```python
from build123d import *

# Parameters (mm, degrees)
SKETCH1_W                      = 57.404
SKETCH1_H                      = 61.214
BOSS_EXTRUDE1_DEPTH            = 1.5875
BOSS_EXTRUDE2_DEPTH            = 1.5875
BOSS_EXTRUDE3_DEPTH            = 54.229
BOSS_EXTRUDE4_DEPTH            = 1.5875
SKETCH6_W                      = 1.63195
SKETCH6_H                      = 1.5875
F_4_CLEARANCE_HOLE1_AT_2_COUNT = 2
F_4_CLEARANCE_HOLE1_AT_2_PITCH = 54.864


with BuildPart() as part:
    # Sketch1 → Boss-Extrude1 (new body)
    with BuildSketch(Plane(origin=(0, 0, 0), x_dir=(1, 0, 0), z_dir=(0, 1, 0))):
        with Locations((28.702, -30.607)):
            Rectangle(SKETCH1_W, SKETCH1_H)
    extrude(amount=BOSS_EXTRUDE1_DEPTH)

    # Sketch2 → Boss-Extrude2 (add)
    with BuildSketch(Plane(origin=(57.404, 0, 0), x_dir=(0, 0, -1), z_dir=(1, 0, 0))):
        with BuildLine():
            Line((-61.214, 1.5875), (0, 1.5875))
            Line((0, 1.5875), (0, 9.144))
            ThreePointArc((0, 9.144), (-1.859871939, 13.634128061), (-6.35, 15.494))
            Line((-6.35, 15.494), (-54.864, 15.494))
            ThreePointArc((-54.864, 15.494), (-59.354128061, 13.634128061), (-61.214, 9.144))
            Line((-61.214, 9.144), (-61.214, 1.5875))
        make_face()
    extrude(amount=-BOSS_EXTRUDE2_DEPTH)

    # Sketch3 → Boss-Extrude3 (add)
    with BuildSketch(Plane.ZY.offset(-55.8165)):
        with BuildLine():
            Line((1.5875, 1.5875), (1.5875, 3.175))
            Line((1.5875, 3.175), (1.5875, 9.144))
            ThreePointArc((1.5875, 9.144), (2.982403955, 12.511596045), (6.35, 13.9065))
            Line((6.35, 13.9065), (6.35, 15.494))
            ThreePointArc((6.35, 15.494), (1.859871939, 13.634128061), (0, 9.144))
            Line((0, 9.144), (0, 1.5875))
            Line((0, 1.5875), (1.5875, 1.5875))
        make_face()
        with BuildLine():
            Line((59.6265, 9.144), (59.6265, 3.175))
            Line((59.6265, 3.175), (59.6265, 1.5875))
            Line((59.6265, 1.5875), (61.214, 1.5875))
            Line((61.214, 1.5875), (61.214, 9.144))
            ThreePointArc((61.214, 9.144), (59.354128061, 13.634128061), (54.864, 15.494))
            Line((54.864, 15.494), (54.864, 13.9065))
            ThreePointArc((54.864, 13.9065), (58.231596045, 12.511596045), (59.6265, 9.144))
        make_face()
    extrude(amount=BOSS_EXTRUDE3_DEPTH)

    # Sketch4 → Boss-Extrude4 (add)
    with BuildSketch(Plane.ZY.offset(-1.5875)):
        with BuildLine():
            Line((0, 0), (61.214, 0))
            Line((61.214, 0), (61.214, 9.144))
            ThreePointArc((61.214, 9.144), (59.354128061, 13.634128061), (54.864, 15.494))
            Line((54.864, 15.494), (6.35, 15.494))
            ThreePointArc((6.35, 15.494), (1.859871939, 13.634128061), (0, 9.144))
            Line((0, 9.144), (0, 0))
        make_face()
    extrude(amount=BOSS_EXTRUDE4_DEPTH)

    # Sketch6 → #4 Clearance Hole1 (revolve, cut)
    with BuildSketch(Plane(origin=(28.575, 1.5875, 58.039), x_dir=(0, 0, 1), z_dir=(1, 0, 0))):
        with Locations((0.815975, 0.79375)):
            Rectangle(SKETCH6_W, SKETCH6_H)
    f_4_clearance_hole1 = revolve(axis=Axis((28.575, 7.9375, 58.039), (0, -1, 0)), mode=Mode.SUBTRACT)

    # #4 Clearance Hole1 at 2: #4 Clearance Hole1 ×2
    with Locations(*[(0, 0, -i * F_4_CLEARANCE_HOLE1_AT_2_PITCH) for i in range(1, F_4_CLEARANCE_HOLE1_AT_2_COUNT)]):
        add(f_4_clearance_hole1, mode=Mode.SUBTRACT)


solid = part.part
```
Source: CAD feature listing. Evaluate the final solid. Frame: model axes, mm. A direction names the side the tool comes from. Coordinates: 2 decimals unless noted, no trailing zeros. Loops run counter-clockwise (first coordinate to the right, second up) from the corner with the lowest first, then second, coordinate; pieces in that order, holes last. Notation, with made-up numbers: M 42,54 L 79,54 A27 cw 79,93 Z; hole C -20,21.25 d1. An arc over 180 degrees is marked long. Use a Markdown table: item, result. Add a question column.
Q1. First-contact query: pin 1 (1 mm diameter, centred on x = 50.5, z = 9, fed in from +Y); pin 2 (1.7 mm diameter, centred on x = 26, y = 14.5, fed in from +Z); pin 3 (4 mm diameter, centred on x = 28.575, z = 3.175, fed in from +Y); pin 4 (1 mm diameter, centred on x = 16.5, z = 36, fed in from -Y). Flat tips, straight axial feed; report the tip coordinate or a pass-through.
Q2. Section query A-A, the plane z = 15. Return loops of the section in (x, y), and give its area (3 significant figures).
Q3. Material intervals for L1, parallel to X at y = 11.25, z = 35.5; L2, parallel to Z at x = 49, y = 7.75; L3, parallel to Y at x = 40, z = 14, sorted ascending.
Q4. Section query D-D, the plane y = 11.75. Return loops of the section in (x, z).
Q5. Draft query along Y for faces 5 (the flat face through (57, 15.494, 30)), 6 (the cylindrical face through (29.08, 12.55, 58.19)), 7 (the flat face through (29, 15, 6.35)). Return one class per face: pulls with the +Y half, pulls with the -Y half, needs draft (parallel to the pull), parting line crosses it, or undercut.
Q6. Section query B-B, the plane y = 3.5. Return loops of the section in (x, z).
Q7. Access query for faces 1 (the cylindrical face through (28.1, 0.8, 59.6)), 2 (the flat face through (29, 5, 0)), 3 (the flat face through (29, 5, 61.214)), 4 (the flat face through (1.588, 9, 30)). Directions: +Z, -Z, +X, -X, +Y, -Y. A direction counts if a zero-diameter tool reaches every point of the face in a straight line with its end or side. Return the directions, or none.
Result:
| question | item | result |
|---|---|---|
| 1 | pin 1 | stops at y = 1.59 |
| 1 | pin 2 | stops at z = 59.34 |
| 1 | pin 3 | stops at y = 15.38 |
| 1 | pin 4 | stops at y = 0 |
| 2 | outline | M 0,0 L 57.4,0 L 57.4,15.49 L 55.82,15.49 L 55.82,1.59 L 1.59,1.59 L 1.59,15.49 L 0,15.49 Z |
| 2 | area | 135 mm2 |
| 3 | L1 | x = 0 to 1.59, 55.82 to 57.4 |
| 3 | L2 | z = 0 to 1.59, 59.63 to 61.21 |
| 3 | L3 | y = 0 to 1.59 |
| 4 | outline | M 0,0.56 L 57.4,0.56 L 57.4,60.65 L 0,60.65 Z; hole M 1.59,2.36 L 55.82,2.36 L 55.82,58.85 L 1.59,58.85 Z |
| 5 | face 5 | pulls with the +Y half |
| 5 | face 6 | undercut |
| 5 | face 7 | needs draft |
| 6 | outline | M 0,0 L 57.4,0 L 57.4,61.21 L 0,61.21 Z; hole M 1.59,1.59 L 55.82,1.59 L 55.82,59.63 L 1.59,59.63 Z |
| 7 | face 1 | -Y |
| 7 | face 2 | -Z, +X, -X, +Y, -Y |
| 7 | face 3 | +Z, +X, -X, +Y, -Y |
| 7 | face 4 | none |
